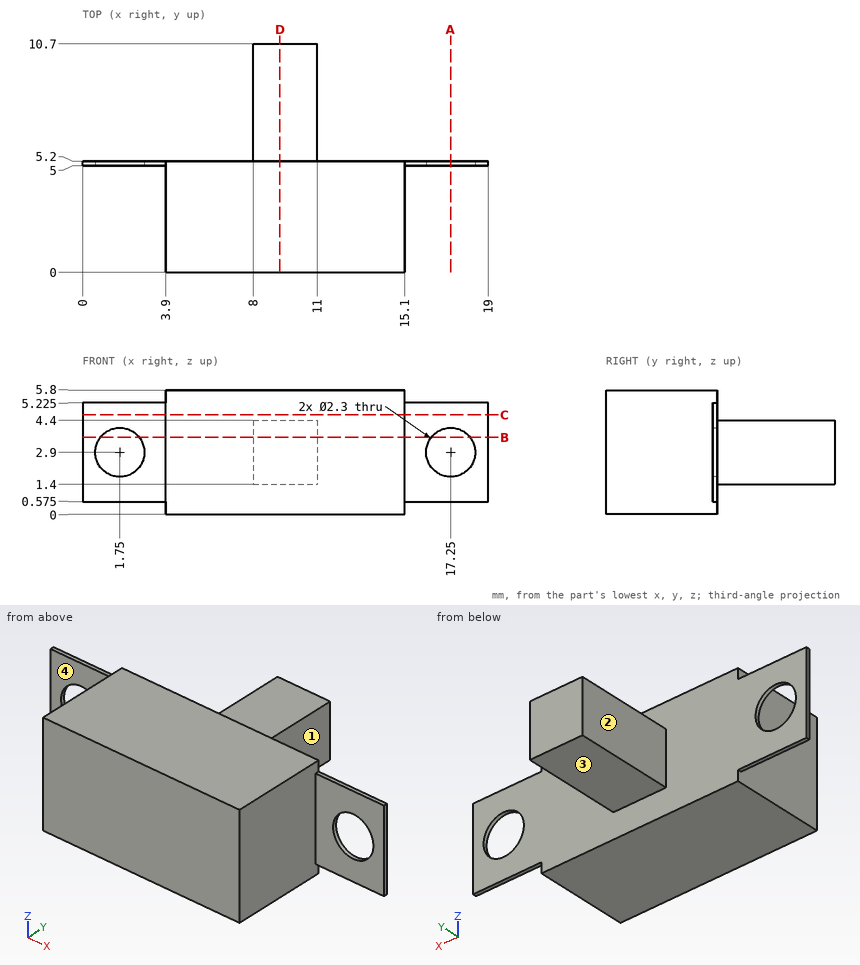
Input: dimensioned drawing with shaded views. Units: mm. Origin: part minimum x, y, z. A direction names the side the tool comes from. Round coordinates to 2 decimals unless told otherwise and drop trailing zeros. Order: outer loops, then holes, each group sorted by start corner. A loop starts at its lowest first (then second) coordinate and runs counter-clockwise, first axis right, second up. Notation, with made-up numbers: (4, 30) - (54, 30) arc R18 ccw to (54, 34) - close; hole circle Ø5 at (15.25, 60.5). An arc over 180 degrees is marked (long way). Answer as a JSON object with one key per item and string values. Group by question number.
(1) Reachability of the marked faces 1, 2, 3 and 4 from +Z, -Z, +X, -X, +Y, -Y: full face, straight path, thin tool, end or side. Return the list, or none.
(2) Cut plane C-C (z = 4.65). Return loops of the section in (x, y).
(3) Cut plane D-D (x = 9.25). Return loops of the section in (y, z), then the cut area to 3 significant figures.
(4) Material intervals for probe 1 along X at (y, z) = (5.15, 2.9); probe 2 along Y at (x, z) = (9, 4.6); probe 3 along X at (y, z) = (1.75, 1.85), sorted ascending. Write a range as from..to.
(5) Pin query (flat end, axial travel): P1, Ø2, axis at x = 17, z = 2, coming from the -Y side; P2, Ø2, axis at y = 9.5, z = 4.5, coming from the -X side; P3, Ø0.9, axis at x = 10, y = 8, coming from the +Z side. Return the tip coordinate at first contact, or that it passes through.
(6) Cut plane A-A (x = 17.25). Return loops of the section in (y, z) (3 decimals).
(7) Cut plane B-B (z = 3.6). Return loops of the section in (x, y), then the cut area to 3 significant figures.
Here are the results:
{
 "1": {"face 1": "+Z, -Z, +X, +Y", "face 2": "+Z, -Z, -X, +Y", "face 3": "-Z, +X, -X, +Y", "face 4": "+Z, -Z, -X, -Y"},
 "2": {"outline": "(0, 5) - (3.9, 5) - (3.9, 0) - (15.1, 0) - (15.1, 5) - (19, 5) - (19, 5.2) - (0, 5.2) - close"},
 "3": {"outline": "(0, 0) - (5.2, 0) - (5.2, 1.4) - (10.7, 1.4) - (10.7, 4.4) - (5.2, 4.4) - (5.2, 5.8) - (0, 5.8) - close", "area": "46.7 mm^2"},
 "4": {"probe 1": "x = 0..0.6, 2.9..16.1, 18.4..19", "probe 2": "y = 0..5.2", "probe 3": "x = 3.9..15.1"},
 "5": {"P1": "stops at y = 5", "P2": "stops at x = 8", "P3": "stops at z = 4.4"},
 "6": {"outline": "(5, 0.575) - (5.2, 0.575) - (5.2, 1.75) - (5, 1.75) - close; (5, 4.05) - (5.2, 4.05) - (5.2, 5.225) - (5, 5.225) - close"},
 "7": {"outline": "(0, 5) - (0.84, 5) - (0.84, 5.2) - (0, 5.2) - close; (2.66, 5) - (3.9, 5) - (3.9, 0) - (15.1, 0) - (15.1, 5) - (16.34, 5) - (16.34, 5.2) - (11, 5.2) - (11, 10.7) - (8, 10.7) - (8, 5.2) - (2.66, 5.2) - close; (18.16, 5) - (19, 5) - (19, 5.2) - (18.16, 5.2) - close", "area": "75.6 mm^2"}
}
